Drawing for the job (mm, zero at the part's lowest x, y, z). Coordinates: 2 decimals unless noted, no trailing zeros. Write each loop counter-clockwise with the first axis right and the second up, starting at its lowest first coordinate (ties: lowest second). Pieces come first, ordered by that corner, then holes. Notation, with made-up numbers: (68, 29) -> (111, 29) arc R20 cw to (111, 35) -> close; hole circle Ø1 at (-26.5, 14.5). An arc over 180 degrees is marked (long way). Answer as CSV lines item,"result".
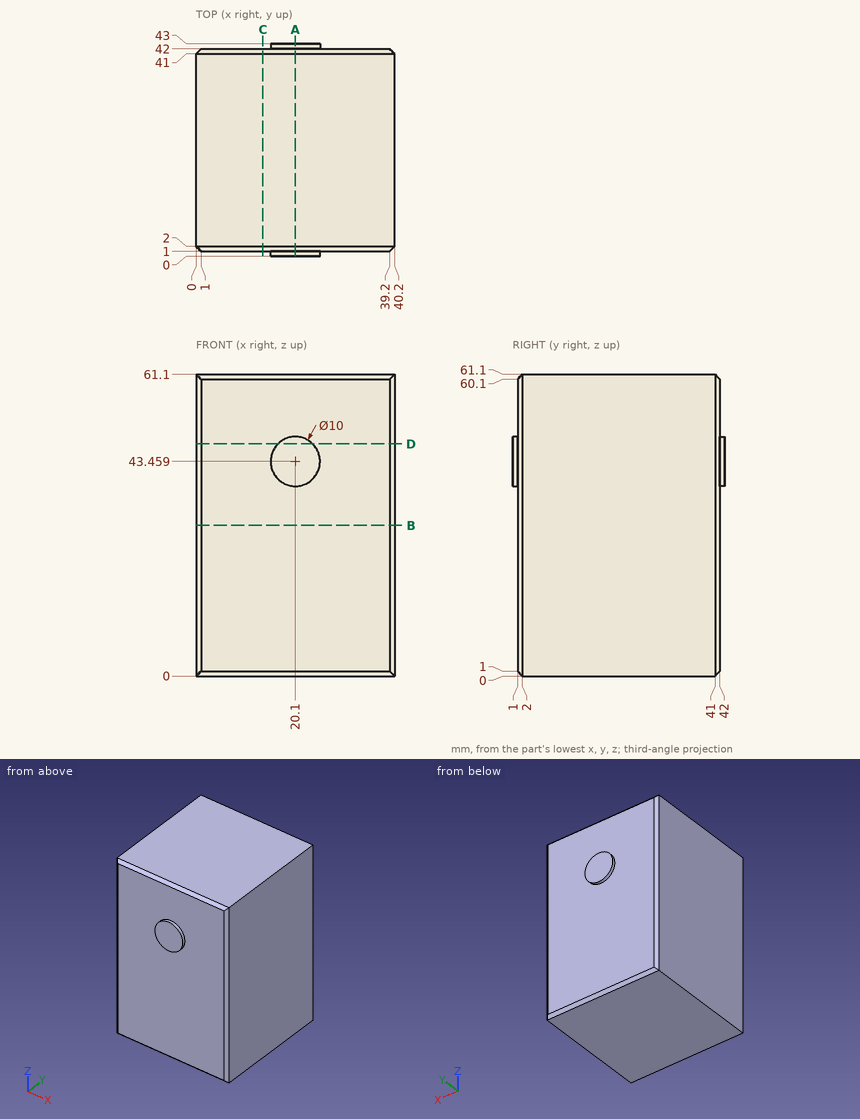
Item 1: Saw through at C-C on x = 13.5. Give the cut face in (y, z), and give its area (3 significant figures).
Answer below:
outline,"(1, 1) -> (2, 0) -> (41, 0) -> (42, 1) -> (42, 60.1) -> (41, 61.1) -> (2, 61.1) -> (1, 60.1) -> close"
area,"2,500 mm2"
Item 2: Wall check: line 1 (Y direction, x = 31, z = 53). Give the ranges that are in metal, low to high. Write a range as from..to.
Answer below:
line 1,"y = 1..42"
Item 3: Saw through at D-D on z = 47. Give the cut face in (x, y), and give its area (3 significant figures).
Answer below:
outline,"(0, 2) -> (1, 1) -> (16.57, 1) -> (16.57, 0) -> (23.63, 0) -> (23.63, 1) -> (39.2, 1) -> (40.2, 2) -> (40.2, 41) -> (39.2, 42) -> (23.63, 42) -> (23.63, 43) -> (16.57, 43) -> (16.57, 42) -> (1, 42) -> (0, 41) -> close"
area,"1,660 mm2"
Item 4: Saw through at A-A on x = 20.1. Give the cut face in (y, z), and give its area (3 significant figures).
Answer below:
outline,"(0, 38.46) -> (1, 38.46) -> (1, 1) -> (2, 0) -> (41, 0) -> (42, 1) -> (42, 38.46) -> (43, 38.46) -> (43, 48.46) -> (42, 48.46) -> (42, 60.1) -> (41, 61.1) -> (2, 61.1) -> (1, 60.1) -> (1, 48.46) -> (0, 48.46) -> close"
area,"2,520 mm2"
Item 5: Saw through at B-B on z = 30.5. Give the cut face in (x, y), and give its area (3 significant figures).
Answer below:
outline,"(0, 2) -> (1, 1) -> (39.2, 1) -> (40.2, 2) -> (40.2, 41) -> (39.2, 42) -> (1, 42) -> (0, 41) -> close"
area,"1,650 mm2"
Item 6: Flat gauge pins, fed straight in: pin 1 (5 mm diameter, centred on x = 33.5, z = 38.5, fed in from +Y); pin 2 (11.5 mm diameter, centred on x = 29, z = 21.5, fed in from -Y). Where does each tip first touch, or does it go through?
Answer below:
pin 1,"stops at y = 42"
pin 2,"stops at y = 1"
